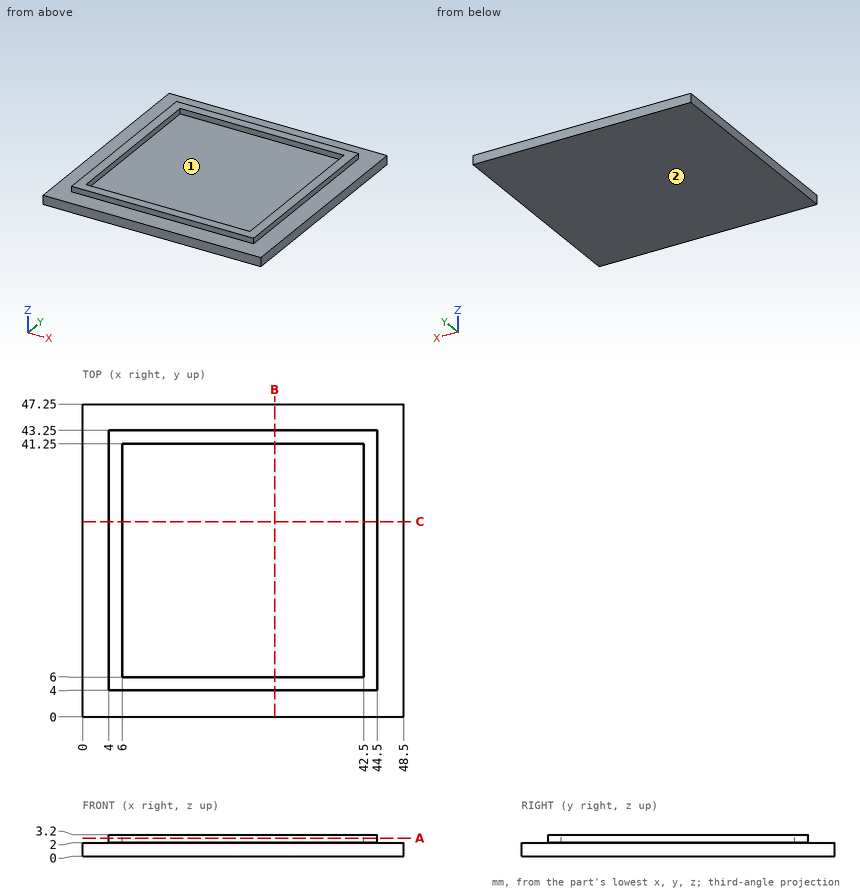
Check sheet for the drawn part. Datum: minimum x, y, z corner. Units: mm. A direction names the side the tool comes from. Round coordinates to 2 decimals unless told otherwise and drop trailing zeros. Write each loop counter-clockwise with the first axis right and the second up, starting at its lowest first coordinate (ties: lowest second). Pieces come first, ordered by that corner, then holes. Notation, with made-up numbers: (75, -10.5) -> (79, -10.5) arc R24 ccw to (79, 4.5) -> close; hole circle Ø11 at (-0.75, 82.25). An arc over 180 degrees is marked (long way). One line per item, written item: value. Start each with the question number.
(1) Cross-section at B-B, the plane x = 29. Record the cut outline in (y, z).
(2) Cross-section at A-A, the plane z = 2.7. Record the cut outline in (x, y), and give its area (3 significant figures).
(3) Cross-section at C-C, the plane y = 29.5. Record the cut outline in (x, z), and give its area (3 significant figures).
(4) Access from +Z, -Z, +X, -X, +Y, -Y to the whole of each face (thin tool, end or side, straight path). Record for the marked faces 1 and 2.
(5) Go/stop test with flat-tipped pins: pin 1 Ø10 at (x, y) = (16, 14.5) entering from +Z; pin 2 Ø0.6 at (y, z) = (30.5, 2.5) entering from +X; pin 3 Ø0.6 at (x, z) = (23, 2.5) entering from -Y. Record where each tip stops, or that it passes through.
(6) Scan lines: line 1 (Y direction, x = 17.5, z = 2.05); line 2 (X direction, y = 13, z = 2.7); line 3 (Z direction, x = 11.5, y = 45.5). Record each from-to range of solid material in increasing order. Write a range as [from, to].
Answer:
1. outline: (0, 0) -> (47.25, 0) -> (47.25, 2) -> (43.25, 2) -> (43.25, 3.2) -> (41.25, 3.2) -> (41.25, 2) -> (6, 2) -> (6, 3.2) -> (4, 3.2) -> (4, 2) -> (0, 2) -> close
2. outline: (4, 4) -> (44.5, 4) -> (44.5, 43.25) -> (4, 43.25) -> close; hole (6, 6) -> (42.5, 6) -> (42.5, 41.25) -> (6, 41.25) -> close
2. area: 303 mm²
3. outline: (0, 0) -> (48.5, 0) -> (48.5, 2) -> (44.5, 2) -> (44.5, 3.2) -> (42.5, 3.2) -> (42.5, 2) -> (6, 2) -> (6, 3.2) -> (4, 3.2) -> (4, 2) -> (0, 2) -> close
3. area: 102 mm²
4. face 1: +Z
4. face 2: -Z, +X, -X, +Y, -Y
5. pin 1: z = 2
5. pin 2: x = 44.5
5. pin 3: y = 4
6. line 1: [4, 6], [41.25, 43.25]
6. line 2: [4, 6], [42.5, 44.5]
6. line 3: [0, 2]
